Here's the drawing with two shaded views (mm, measured from the low corner). I have some questions. Round coordinates to 2 decimals unless told otherwise and drop trailing zeros. Loops run counter-clockwise (first coordinate to the right, second up) from the corner with the lowest first, then second, coordinate; pieces in that order, holes last. Notation, with made-up numbers: M 85,23 L 139,23 A21 ccw 139,28 Z; hole C -9,-39.75 d7. An arc over 180 degrees is marked long. Answer as CSV lines item,"result".
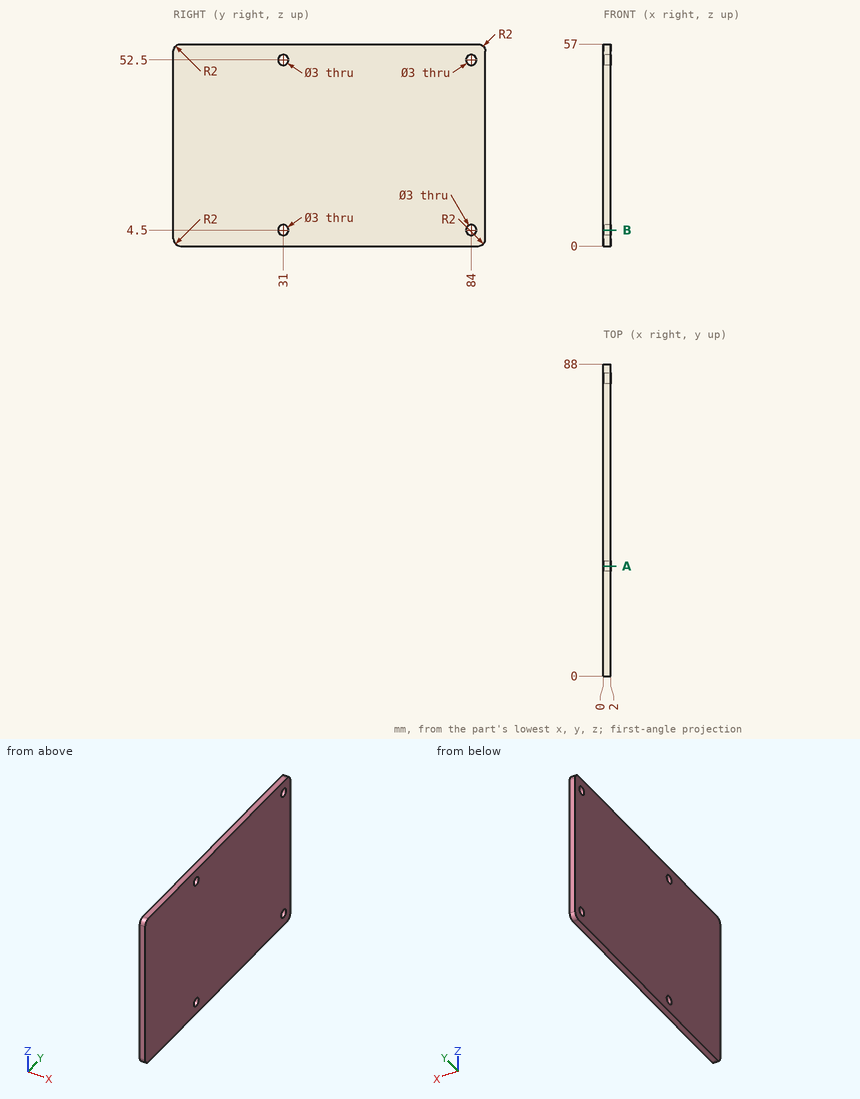
1. For P1, Ø8, axis at y = 46, z = 31.5, coming from the -X side; P2, Ø1.8, axis at y = 31, z = 4.5, coming from the +X side, each with a flat end and sliding along its axis, tell me the tip position at first contact or that it passes through.
Evaluation:
P1,"stops at x = 0"
P2,"passes through"
2. If I drill on line 1 (Z direction, x = 0.7, y = 84); line 2 (Y direction, x = 0.5, z = 5), over which ranges is the centre line in solid material (lowest first)? Write a range as [from, to].
Evaluation:
line 1,"z = [0, 3], [6, 51], [54, 57]"
line 2,"y = [0, 29.59], [32.41, 82.59], [85.41, 88]"
3. I want a section at A-A, the plane y = 31. Please give me the cut outline in (x, z).
Evaluation:
outline,"M 0,0 L 2,0 L 2,3 L 0,3 Z; M 0,6 L 2,6 L 2,51 L 0,51 Z; M 0,54 L 2,54 L 2,57 L 0,57 Z"
4. I want a section at B-B, the plane z = 4.5. Please give me the cut outline in (x, y).
Evaluation:
outline,"M 0,0 L 2,0 L 2,29.5 L 0,29.5 Z; M 0,32.5 L 2,32.5 L 2,82.5 L 0,82.5 Z; M 0,85.5 L 2,85.5 L 2,88 L 0,88 Z"
